Autodesk Fusion 360 part; units mm, degrees
sketch "Sketch1" plane through (0, 0, 0) normal (0, 0, 1) x (1, 0, 0)
  circle A0 centre (0, 0) radius 20
  dimension "d1" = 40
ref_plane "WorkPlane1" through (0, 0, 30) normal (0, 0, 1) x (1, 0, 0)
sketch "Sketch2" plane through (0, 0, 30) normal (0, 0, 1) x (1, 0, 0)
  circle A0 centre (0, 0) radius 15
  dimension "d3" = 30
loft "Loft1" add profiles "Sketch2", "Sketch1" section 1 section 2
sketch "Sketch3" plane through (0, 0, 0) normal (0, 0, -1) x (1, 0, 0)
  circle A0 centre (0, 0) radius 20
  circle A1 centre (0, 0) radius 7.5
  dimension "d4" = 15
extrude "Extrude1" cut sketch "Sketch3" against normal blind 27 contours A1
sketch "Sketch4" plane through (0, 0, 27) normal (0, 0, -1) x (1, 0, 0)
  circle A0 centre (0, 0) radius 7.5
  circle A1 centre (0, 0) radius 3
  dimension "d7" = 6
extrude "Extrude2" cut sketch "Sketch4" against normal blind 7 contours A1
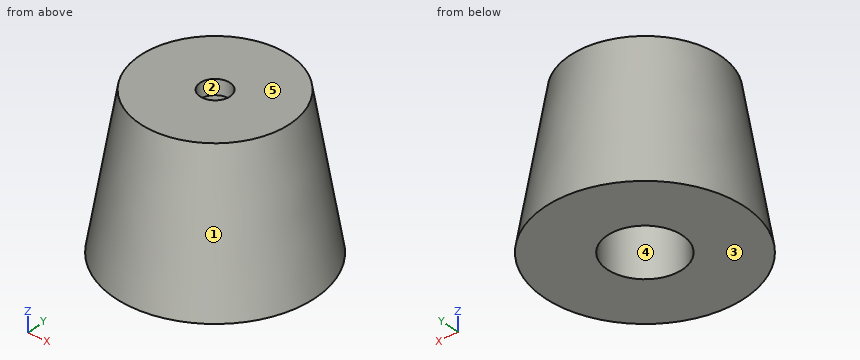
The model under review builds one solid part; all positions refer to its coordinate system, in mm. Face numbers are marked on the shaded views. A direction names the side the tool comes from. Round coordinates to 2 decimals unless told otherwise and drop trailing zeros. Order: outer loops, then holes, each group sorted by start corner. A loop starts at its lowest first (then second) coordinate and runs counter-clockwise, first axis right, second up. Notation, with made-up numbers: (54.5, 17.25) - (113.5, 17.25) arc R19 cw to (113.5, 51.25) - close; hole circle Ø7 at (-20, 37.5). An arc over 180 degrees is marked (long way). Use one line per item in the form item = value.
Q1. Add section B-B on z = 15. Give the boundary of the cut face in (x, y), then the cut area to 3 significant figures.
Response values:
outline = circle Ø35 at (0, 0); hole circle Ø15 at (0, 0)
area = 785 mm^2
Q2. Clearance check with flat-ended pins moving along their axes: P1, Ø4, axis at y = -8.5, z = 5, coming from the +X side; P2, Ø2, axis at x = 5, z = 3.5, coming from the +Y side; P3, Ø8, axis at y = -2, z = 9.5, coming from the -X side. State where each tip first meets the part, or that it passes through.
Response values:
P1 = 18.11
P2 = 19.06
P3 = -19.04
Q3. To check wall thickness, follow line 1 (Y direction, x = 0, z = 8); line 2 (Y direction, x = 0, z = 13); line 3 (X direction, y = 2, z = 12). State the ranges of each line that lie inside material, in increasing order.
Response values:
line_1 = -18.67 to -7.5, 7.5 to 18.67
line_2 = -17.83 to -7.5, 7.5 to 17.83
line_3 = -17.89 to -7.23, 7.23 to 17.89
Q4. Add section A-A on x = 0. Give the boundary of the cut face in (y, z), then the cut area to 3 significant figures.
Response values:
outline = (-20, 0) - (-7.5, 0) - (-7.5, 27) - (-3, 27) - (-3, 30) - (-15, 30) - close; (3, 27) - (7.5, 27) - (7.5, 0) - (20, 0) - (15, 30) - (3, 30) - close
area = 627 mm^2
Q5. Add section C-C on z = 2. Give the boundary of the cut face in (x, y).
Response values:
outline = circle Ø39.33 at (0, 0); hole circle Ø15 at (0, 0)
Q6. Tool access review of the marked faces 4 and 5: name each direction out of +Z, -Z, +X, -X, +Y, -Y from which nothing blocks a thin tool from reaching the whole face with its end or side.
Response values:
face_4 = -Z
face_5 = +Z, +X, -X, +Y, -Y
Q7. Mouldability with a two-part tool opening along Y and no side actions: class the marked faces 1, 2 and 3 as pulls with the +Y half, pulls with the -Y half, needs draft (parallel to the pull), parting line crosses it, or undercut.
Response values:
face_1 = parting line crosses it
face_2 = undercut
face_3 = needs draft
